Read the model definition and answer for the solid it produces. Units are mm, in the model's axes. A direction names the side the tool comes from. Coordinates: 2 decimals unless noted, no trailing zeros. Write each loop counter-clockwise with the first axis right and the second up, starting at its lowest first coordinate (ties: lowest second). Pieces come first, ordered by that corner, then holes.
1) The part is cut by section D-D (x = 39). Determine the outline of the cut face in (y, z), then the cut area to 3 significant figures.
2) Determine the mould class of faces 1 (the face through (21, -1, -12.7)), 2 (the face through (21, 1, 12.7)), 3 (the face through (90, 30, 5.08)), 4 (the face through (-46.97, -54.2, -0.18)) for opening direction Z: +Z half, -Z half, draft (parallel to the pull), parting line (faces both ways), or undercut.
3) Each of these flat-tipped pins is pushed along its axis until it touches: pin 1 Ø7 at (x, z) = (0, 1.5) entering from -Y; pin 2 Ø5 at (x, z) = (-44.5, -5) entering from +Y; pin 3 Ø2 at (x, z) = (61.5, 3.5) entering from -Y; pin 4 Ø17 at (x, y) = (-44.9, 44.9) entering from +Z. Where does it stop, or does it pass through?
4) Find the intervals of material crossed by line 1 (Y direction, x = 0, z = 3); line 2 (Y direction, x = 0, z = -6.75); line 3 (Y direction, x = -37, z = -5), in increasing order.
5) Which of the six approach directions +Z, -Z, +X, -X, +Y, -Y give full straight-line access (tool end or side, diameter ignored) to faces 5 (the face through (-3.175, 7, 0)), 6 (the face through (90, -30, -5.08))?
6) The part is cut by section A-A (y = 0). Determine the outline of the cut face in (x, z), then the cut area to 3 significant figures.
7) The part is cut by section B-B (x = 0). Determine the outline of the cut face in (y, z), then the cut area to 3 significant figures.
8) The part is cut by section C-C (y = -63.5). Determine the outline of the cut face in (x, z), then the cut area to 3 significant figures.
from build123d import *

# Parameters (mm, degrees)
CUT_EXTRUDE1_DEPTH      = 145.244271983
CUT_EXTRUDE1_DEPTH_BACK = 145.244271983
SKETCH5_R               = 19.05
SKETCH5_R_2             = 9.525
CUT_EXTRUDE5_DEPTH      = 145.244271983
CUT_EXTRUDE5_DEPTH_BACK = 145.244271983
SKETCH6_R               = 5.588
CUT_EXTRUDE6_DEPTH      = 145.244271983
CUT_EXTRUDE6_DEPTH_BACK = 145.244271983
SKETCH8_W               = 6.35
SKETCH8_H               = 5.561617784


with BuildPart() as part:
    # Sketch1 → Revolve2 (revolve)
    with BuildSketch(Plane(origin=(0, 0, 0), x_dir=(0, 0, -1), z_dir=(1, 0, 0))):
        Polygon((0, 0), (-12.7, 0), (-12.7, 101.6), (-5.08, 101.6), (-5.08, 93.98), (5.08, 93.98), (5.08, 101.6), (12.7, 101.6), (12.7, 0), align=None)
    revolve(axis=Axis((0, 0, 0), (0, 0, 1)))

    # Sketch5 → Cut-Extrude1 (cut, two sides: drawn at the far end of the back side and taken through both)
    with BuildSketch(Plane.XY.offset(-CUT_EXTRUDE1_DEPTH_BACK)):
        with Locations((0, -63.5)):
            Circle(SKETCH5_R)
        with Locations((44.901280605, -44.901280605)):
            Circle(SKETCH5_R_2)
        with Locations((-63.5, 0)):
            Circle(SKETCH5_R)
        with Locations((-44.901280605, -44.901280605)):
            Circle(SKETCH5_R_2)
        with Locations((0, 63.5)):
            Circle(SKETCH5_R)
        with Locations((-44.901280605, 44.901280605)):
            Circle(SKETCH5_R_2)
        with Locations((63.5, 0)):
            Circle(SKETCH5_R)
        with Locations((44.901280605, 44.901280605)):
            Circle(SKETCH5_R_2)
    extrude(amount=CUT_EXTRUDE1_DEPTH + CUT_EXTRUDE1_DEPTH_BACK, mode=Mode.SUBTRACT)

    # Sketch6 → Cut-Extrude5 (cut, two sides: drawn at the far end of the back side and taken through both)
    with BuildSketch(Plane.XY.offset(-CUT_EXTRUDE5_DEPTH_BACK)):
        Circle(SKETCH6_R)
    extrude(amount=CUT_EXTRUDE5_DEPTH + CUT_EXTRUDE5_DEPTH_BACK, mode=Mode.SUBTRACT)

    # Sketch8 → Cut-Extrude6 (cut, two sides: drawn at the far end of the back side and taken through both)
    with BuildSketch(Plane.XY.offset(-CUT_EXTRUDE6_DEPTH_BACK)):
        with Locations((0, 7.379191108)):
            Rectangle(SKETCH8_W, SKETCH8_H)
    extrude(amount=CUT_EXTRUDE6_DEPTH + CUT_EXTRUDE6_DEPTH_BACK, mode=Mode.SUBTRACT)


solid = part.part
Reported:
1. outline: (-93.82, -12.7) - (-52.38, -12.7) - (-52.38, 12.7) - (-93.82, 12.7) - (-93.82, 5.08) - (-85.51, 5.08) - (-85.51, -5.08) - (-93.82, -5.08) - close; (-37.42, -12.7) - (37.42, -12.7) - (37.42, 12.7) - (-37.42, 12.7) - close; (52.38, -12.7) - (93.82, -12.7) - (93.82, -5.08) - (85.51, -5.08) - (85.51, 5.08) - (93.82, 5.08) - (93.82, 12.7) - (52.38, 12.7) - close
1. area: 3,840 mm2
2. face 1: -Z half
2. face 2: +Z half
2. face 3: undercut
2. face 4: draft
3. pin 1: stops at y = -93.98
3. pin 2: stops at y = 92.51
3. pin 3: stops at y = -71.92
3. pin 4: passes through
4. line 1: y = -93.98 to -82.55, -44.45 to -5.59, 10.16 to 44.45, 82.55 to 93.98
4. line 2: y = -101.6 to -82.55, -44.45 to -5.59, 10.16 to 44.45, 82.55 to 101.6
4. line 3: y = -86.39 to -50.22, -39.58 to 39.58, 50.22 to 86.39
5. face 5: +Z, -Z
5. face 6: none
6. outline: (-101.6, -12.7) - (-82.55, -12.7) - (-82.55, 12.7) - (-101.6, 12.7) - (-101.6, 5.08) - (-93.98, 5.08) - (-93.98, -5.08) - (-101.6, -5.08) - close; (-44.45, -12.7) - (-5.59, -12.7) - (-5.59, 12.7) - (-44.45, 12.7) - close; (5.59, -12.7) - (44.45, -12.7) - (44.45, 12.7) - (5.59, 12.7) - close; (82.55, -12.7) - (101.6, -12.7) - (101.6, -5.08) - (93.98, -5.08) - (93.98, 5.08) - (101.6, 5.08) - (101.6, 12.7) - (82.55, 12.7) - close
6. area: 2,790 mm2
7. outline: (-101.6, -12.7) - (-82.55, -12.7) - (-82.55, 12.7) - (-101.6, 12.7) - (-101.6, 5.08) - (-93.98, 5.08) - (-93.98, -5.08) - (-101.6, -5.08) - close; (-44.45, -12.7) - (-5.59, -12.7) - (-5.59, 12.7) - (-44.45, 12.7) - close; (10.16, -12.7) - (44.45, -12.7) - (44.45, 12.7) - (10.16, 12.7) - close; (82.55, -12.7) - (101.6, -12.7) - (101.6, -5.08) - (93.98, -5.08) - (93.98, 5.08) - (101.6, 5.08) - (101.6, 12.7) - (82.55, 12.7) - close
7. area: 2,670 mm2
8. outline: (-79.31, -12.7) - (-19.05, -12.7) - (-19.05, 12.7) - (-79.31, 12.7) - (-79.31, 5.08) - (-69.28, 5.08) - (-69.28, -5.08) - (-79.31, -5.08) - close; (19.05, -12.7) - (79.31, -12.7) - (79.31, -5.08) - (69.28, -5.08) - (69.28, 5.08) - (79.31, 5.08) - (79.31, 12.7) - (19.05, 12.7) - close
8. area: 2,860 mm2
